from build123d import *

# Parameters (mm, degrees)
ESQUISSE1_W                     = 80
ESQUISSE1_H                     = 80
BOSS_EXTRU_1_DEPTH              = 5
ESQUISSE2_W                     = 5
ESQUISSE2_H                     = 5
BOSS_EXTRU_2_DEPTH              = 5
R_P_TITION_LIN_AIRE1_COUNT      = 2
R_P_TITION_LIN_AIRE1_PITCH      = 85
R_P_TITION_LIN_AIRE1_COUNT_DIR2 = 8
R_P_TITION_LIN_AIRE1_PITCH_DIR2 = 10
ENL_V_MAT_EXTRU_1_DEPTH         = 10
ESQUISSE9_W                     = 5
ESQUISSE9_H                     = 5
ENL_V_MAT_EXTRU_6_DEPTH         = 10
R_P_TITION_LIN_AIRE4_COUNT      = 2
R_P_TITION_LIN_AIRE4_PITCH      = 10
R_P_TITION_LIN_AIRE4_COL_COUNT  = 2
R_P_TITION_LIN_AIRE4_COL_PITCH  = 10
ENL_V_MAT_EXTRU_7_DEPTH         = 10


with BuildPart() as part:
    # Esquisse1 → Boss.-Extru.1 (new body)
    with BuildSketch(Plane(origin=(0, 0, 0), x_dir=(1, 0, 0), z_dir=(0, 1, 0))):
        Rectangle(ESQUISSE1_W, ESQUISSE1_H)
    extrude(amount=BOSS_EXTRU_1_DEPTH)

    # Esquisse2 → Boss.-Extru.2 (add)
    with BuildSketch(Plane(origin=(0, 5, 0), x_dir=(1, 0, 0), z_dir=(0, 1, 0))):
        with Locations((-42.5, 37.5)):
            Rectangle(ESQUISSE2_W, ESQUISSE2_H)
    boss_extru_2 = extrude(amount=-BOSS_EXTRU_2_DEPTH)

    # Répétition linéaire1: Boss.-Extru.2 2 × 8
    with Locations(*[(i * R_P_TITION_LIN_AIRE1_PITCH, 0, j * R_P_TITION_LIN_AIRE1_PITCH_DIR2) for i in range(R_P_TITION_LIN_AIRE1_COUNT) for j in range(R_P_TITION_LIN_AIRE1_COUNT_DIR2) if (i, j) != (0, 0)]):
        add(boss_extru_2)

    # Esquisse3 → Enlèv. mat.-Extru.1 (cut)
    with BuildSketch(Plane(origin=(0, 5, 0), x_dir=(1, 0, 0), z_dir=(0, 1, 0))):
        Polygon((40, 4.05), (38.25, 4.05), (38.25, 5.55), (35.5, 5.55), (35.5, 4.05), (34, 4.05), (34, 1.3), (35.5, 1.3), (35.5, -0.2), (38.25, -0.2), (38.25, 1.3), (40, 1.3), align=None)
    enl_v_mat_extru_1 = extrude(amount=-ENL_V_MAT_EXTRU_1_DEPTH, mode=Mode.SUBTRACT)

    # Esquisse9 → Enlèv. mat.-Extru.6 (cut)
    with BuildSketch(Plane(origin=(0, 5, 0), x_dir=(1, 0, 0), z_dir=(0, 1, 0))):
        with Locations((7.5, 0)):
            Rectangle(ESQUISSE9_W, ESQUISSE9_H)
    enl_v_mat_extru_6 = extrude(amount=-ENL_V_MAT_EXTRU_6_DEPTH, mode=Mode.SUBTRACT)

    # Répétition linéaire4: Enlèv. mat.-Extru.6 ×2
    with Locations(*[(0, 0, -i * R_P_TITION_LIN_AIRE4_PITCH) for i in range(1, R_P_TITION_LIN_AIRE4_COUNT)]):
        add(enl_v_mat_extru_6, mode=Mode.SUBTRACT)

    # Répétition linéaire4 col: Enlèv. mat.-Extru.6 ×2
    with Locations(*[(0, 0, i * R_P_TITION_LIN_AIRE4_COL_PITCH) for i in range(1, R_P_TITION_LIN_AIRE4_COL_COUNT)]):
        add(enl_v_mat_extru_6, mode=Mode.SUBTRACT)

    # Symétrie3: Enlèv. mat.-Extru.1 across plane
    add(enl_v_mat_extru_1.mirror(Plane(origin=(0, 0, 0), x_dir=(0, 0, 1), z_dir=(1, 0, 0))), mode=Mode.SUBTRACT)

    # Esquisse7 → Enlèv. mat.-Extru.7 (cut)
    with BuildSketch(Plane(origin=(0, 5, 0), x_dir=(1, 0, 0), z_dir=(0, 1, 0))):
        Polygon((-35, 40), (0, 40), (0, 5), (-30, 5), align=None)
        Polygon((-35, -40), (0, -40), (0, -5), (-30, -5), align=None)
    extrude(amount=-ENL_V_MAT_EXTRU_7_DEPTH, mode=Mode.SUBTRACT)


solid = part.part
For this review, take the finished solid that the model builds, in its own axes (mm). A direction names the side the tool comes from. Round coordinates to 2 decimals unless told otherwise and drop trailing zeros. Write each loop counter-clockwise with the first axis right and the second up, starting at its lowest first coordinate (ties: lowest second). Pieces come first, ordered by that corner, then holes. Notation, with made-up numbers: M 27.5,22 L 43.5,22 A30 cw 43.5,54 Z; hole C 37.25,-9 d3. An arc over 180 degrees is marked long. Write item = value, one per line. Start each with the question number.
(1) Clearance check with flat-ended pins moving along their axes: pin 1 Ø2.5 at (x, y) = (43.5, 1.5) entering from +Z; pin 2 Ø1.5 at (y, z) = (4.5, -11.5) entering from +X; pin 3 Ø2.5 at (x, y) = (-8, 1.5) entering from +Z. State where each tip first meets the part, or that it passes through.
(2) We need section B-B (z = -18). Give the boundary of the cut face in (x, y).
(3) For faces 1 (the face through (42, 3, -20)), 2 (the face through (-43, 3, -20)), 3 (the face through (-32.465, 2.535, 22.255)), 4 (the face through (-32.465, 2.535, -22.255)), list the 3-axis set-ups (+Z, -Z, +X, -X, +Y, -Y) from which the entire face can be reached by the end or side of a thin tool; tool diameter is ignored.
(4) We need section D-D (z = 26.5). Give the boundary of the cut face in (x, y), then the cut area to 3 significant figures.
(5) For line 1 along X through (y, z) = (3.7, 9.5); line 2 along Z through (x, y) = (-12, 2.6); line 3 along X through (y, z) = (2.2, 22.5), list the stretches that pass through material, from the lowest coordinate up.
(6) We need section C-C (x = -32.5). Give the boundary of the cut face in (y, z), then the cut area to 3 significant figures.
(7) We need section A-A (x = 8). Give the boundary of the cut face in (y, z), then the cut area to 3 significant figures.
(8) The part is to be moulded in two halves that separate along X. For faces 5 (the face through (7, 3, -7.5)), 6 (the face through (-40, 2, 8)), 7 (the face through (-43, 3, 20)), 8 (the face through (10, 3, 0)), say which applies: +X half, -X half, draft (parallel to the pull), parting line (faces both ways), or undercut.
Results found:
q1.pin_1 = 35
q1.pin_2 = 40
q1.pin_3 = 5
q2.outline = M -45,0 L -31.86,0 L -31.86,5 L -45,5 Z; M 0,0 L 45,0 L 45,5 L 0,5 Z
q3.face_1 = +X, +Y, -Y
q3.face_2 = -X, +Y, -Y
q3.face_3 = +Z, +Y, -Y
q3.face_4 = -Z, +Y, -Y
q4.outline = M -40,0 L -33.07,0 L -33.07,5 L -40,5 Z; M 0,0 L 40,0 L 40,5 L 0,5 Z
q4.area = 235 mm²
q5.line_1 = -40 to -30.64, 0 to 5, 10 to 40
q5.line_2 = -5 to 5
q5.line_3 = -45 to -32.5, 0 to 45
q6.outline = M 0,-22.5 L 5,-22.5 L 5,22.5 L 0,22.5 Z
q6.area = 225 mm²
q7.outline = M 0,-40 L 5,-40 L 5,-12.5 L 0,-12.5 Z; M 0,-7.5 L 5,-7.5 L 5,-2.5 L 0,-2.5 Z; M 0,2.5 L 5,2.5 L 5,7.5 L 0,7.5 Z; M 0,12.5 L 5,12.5 L 5,40 L 0,40 Z
q7.area = 325 mm²
q8.face_5 = undercut
q8.face_6 = -X half
q8.face_7 = draft
q8.face_8 = undercut
